```python
from build123d import *

# Parameters (mm, degrees)
SKETCH1_W           = 79
SKETCH1_H           = 53
BOSS_EXTRUDE1_DEPTH = 2
SKETCH2_R           = 2.5
BOSS_EXTRUDE2_DEPTH = 2.7
SKETCH3_R           = 1.5
BOSS_EXTRUDE3_DEPTH = 1.6
SKETCH5_R           = 0.75
CUT_EXTRUDE1_DEPTH  = 2
SKETCH6_W           = 79
SKETCH6_H           = 53
SKETCH6_W_2         = 75
SKETCH6_H_2         = 49
BOSS_EXTRUDE4_DEPTH = 8
SKETCH7_W           = 77
SKETCH7_H           = 51
SKETCH7_W_2         = 75
SKETCH7_H_2         = 49
BOSS_EXTRUDE5_DEPTH = 1.6
CUT_EXTRUDE2_DEPTH  = 2
FILLET1_R           = 1


with BuildPart() as part:
    # Sketch1 → Boss-Extrude1 (new body)
    with BuildSketch(Plane.XY):
        with Locations((39.5, 26.5)):
            Rectangle(SKETCH1_W, SKETCH1_H)
    extrude(amount=BOSS_EXTRUDE1_DEPTH)

    # Sketch2 → Boss-Extrude2 (add)
    with BuildSketch(Plane.XY.offset(2)):
        with Locations(Location((5, 47.8, 0), (0, 0, 180))):
            Circle(SKETCH2_R)
        with Locations(Location((74, 47.8, 0), (0, 0, 180))):
            Circle(SKETCH2_R)
        with Locations(Location((74, 5.2, 0), (0, 0, 180))):
            Circle(SKETCH2_R)
        with Locations(Location((5, 5.2, 0), (0, 0, 180))):
            Circle(SKETCH2_R)
    extrude(amount=BOSS_EXTRUDE2_DEPTH)

    # Sketch3 → Boss-Extrude3 (add)
    with BuildSketch(Plane.XY.offset(4.7)):
        with Locations((5, 47.8)):
            Circle(SKETCH3_R)
        with Locations((5, 5.2)):
            Circle(SKETCH3_R)
        with Locations((74, 47.8)):
            Circle(SKETCH3_R)
        with Locations((74, 5.2)):
            Circle(SKETCH3_R)
    extrude(amount=BOSS_EXTRUDE3_DEPTH)

    # Sketch5 → Cut-Extrude1 (cut)
    with BuildSketch(Plane.XY.offset(6.3)):
        with Locations((74, 5.2)):
            Circle(SKETCH5_R)
        with Locations((74, 47.8)):
            Circle(SKETCH5_R)
        with Locations((5, 47.8)):
            Circle(SKETCH5_R)
        with Locations((5, 5.2)):
            Circle(SKETCH5_R)
    extrude(amount=-CUT_EXTRUDE1_DEPTH, mode=Mode.SUBTRACT)

    # Sketch6 → Boss-Extrude4 (add)
    with BuildSketch(Plane.XY.offset(2)):
        with Locations((39.5, 26.5)):
            Rectangle(SKETCH6_W, SKETCH6_H)
        with Locations((39.5, 26.5)):
            Rectangle(SKETCH6_W_2, SKETCH6_H_2, mode=Mode.SUBTRACT)
    extrude(amount=BOSS_EXTRUDE4_DEPTH)

    # Sketch7 → Boss-Extrude5 (add)
    with BuildSketch(Plane.XY.offset(10)):
        with Locations((39.5, 26.5)):
            Rectangle(SKETCH7_W, SKETCH7_H)
        with Locations((39.5, 26.5)):
            Rectangle(SKETCH7_W_2, SKETCH7_H_2, mode=Mode.SUBTRACT)
    extrude(amount=BOSS_EXTRUDE5_DEPTH)

    # Sketch8 → Cut-Extrude2 (cut)
    with BuildSketch(Plane.XY.offset(2)):
        with BuildLine():
            Line((46.930127019, 21.4), (62.6, 21.4))
            Line((62.6, 21.4), (62.6, 22.4))
            Line((62.6, 22.4), (46.308099244, 22.4))
            ThreePointArc((46.308099244, 22.4), (38.6, 23.9), (46.308099244, 25.4))
            Line((46.308099244, 25.4), (62.6, 25.4))
            Line((62.6, 25.4), (62.6, 26.4))
            Line((62.6, 26.4), (46.930127019, 26.4))
            ThreePointArc((46.930127019, 26.4), (37.6, 23.9), (46.930127019, 21.4))
        make_face()
    extrude(amount=-CUT_EXTRUDE2_DEPTH, mode=Mode.SUBTRACT)

    # Fillet1
    fillet1_edges = [part.edges().sort_by_distance(p)[0] for p in [
        (39.5, 53, 0),
        (79, 26.5, 0),
        (39.5, 0, 0),
        (0, 26.5, 0),
        (0, 53, 5),
        (79, 53, 5),
        (79, 0, 5),
        (0, 0, 5),
        (1, 52, 10.8),
        (1, 1, 10.8),
        (78, 1, 10.8),
        (78, 52, 10.8),
    ]]
    fillet(fillet1_edges, radius=FILLET1_R)


solid = part.part
```
Can you work these out from the model? Positions are in its coordinate system, mm. A direction names the side the tool comes from. Give positions to 0.01 mm unless a question says otherwise; leave off trailing zeros. Loops run counter-clockwise (first coordinate to the right, second up) from the corner with the lowest first, then second, coordinate; pieces in that order, holes last. Notation, with made-up numbers: M -16.5,42.25 L 7.5,42.25 A12 cw 7.5,56.25 Z; hole C 20.5,21 d4. An arc over 180 degrees is marked long. One line per question, with ' | ' between items. Start each with the question number.
Q1. If we section it at B-B (x = 57): Please give me the cut outline in (y, z), plus the area to 3 significant figures.
Q2. If we mould it in two halves opening along Y, with no side actions, what happens to faces 4 (the cylindrical face through (4.45, 5.71, 5.31)), 5 (the flat face through (55, 22.4, 1)), 6 (the flat face through (39, 53, 5)), 7 (the flat face through (39, 0, 5))? For each: +Y half, -Y half, draft (parallel to the pull), parting line (faces both ways), or undercut.
Q3. If we section it at D-D (x = 13): Please give me the cut outline in (y, z).
Q4. If I drill on line 1 (Y direction, x = 5, z = 4.8); line 2 (Y direction, x = 57, z = 1.5); line 3 (X direction, y = 5, z = 3.75), over which ranges is the centre line in solid material (lowest first)? Write a range as from..to.
Q5. If we section it at A-A (z = 5.5): State how many separate pieces and enclosed holes the cut face has, plus the area to 3 significant figures.
Q6. If we section it at C-C (y = 8.5): Please give me the cut outline in (x, z), plus the area to 3 significant figures.
Q7. For pin 1 Ø2.5 at (x, y) = (73.5, 4.5) entering from +Z; pin 2 Ø24.5 at (x, y) = (31.5, 19) entering from +Z; pin 3 Ø0.8 at (y, z) = (25.5, 0.5) entering from -X (3 decimals), each with a flat end and sliding along its axis, tell me the tip position at first contact or that it passes through.
Q8. For faces 1 (the flat face through (54, 25.4, 1)), 2 (the flat face through (74, 7, 4.7)), 3 (the flat face through (39, 1, 11)), which set-ups out of +Z, -Z, +X, -X, +Y, -Y let a thin tool reach every point of the face, with its end or its side?
Computed:
1) outline: M 0,1 A1 ccw 1,0 L 21.4,0 L 21.4,2 L 2,2 L 2,11.6 L 1,11.6 L 1,10 L 0,10 Z; M 22.4,0 L 25.4,0 L 25.4,2 L 22.4,2 Z; M 26.4,0 L 52,0 A1 ccw 53,1 L 53,10 L 52,10 L 52,11.6 L 51,11.6 L 51,2 L 26.4,2 Z | area: 137 mm²
2) face 4: undercut | face 5: undercut | face 6: +Y half | face 7: -Y half
3) outline: M 0,1 A1 ccw 1,0 L 52,0 A1 ccw 53,1 L 53,10 L 52,10 L 52,11.6 L 51,11.6 L 51,2 L 2,2 L 2,11.6 L 1,11.6 L 1,10 L 0,10 Z
4) line 1: y = 0..2, 3.7..4.45, 5.95..6.7, 46.3..47.05, 48.55..49.3, 51..53 | line 2: y = 0..21.4, 22.4..25.4, 26.4..53 | line 3: x = 0..2, 2.51..7.49, 71.51..76.49, 77..79
5) separate pieces: 5 | enclosed holes: 5 | area: 532 mm²
6) outline: M 0,1 A1 ccw 1,0 L 78,0 A1 ccw 79,1 L 79,10 L 78,10 L 78,11.6 L 77,11.6 L 77,2 L 2,2 L 2,11.6 L 1,11.6 L 1,10 L 0,10 Z | area: 193 mm²
7) pin 1: stops at z = 6.3 | pin 2: stops at z = 2 | pin 3: stops at x = 0.005
8) face 1: +Z, -Z | face 2: +Z | face 3: +Z, +X, -X, -Y
